Part model, mm, in its own coordinate system. Face numbers are marked on the shaded views. Coordinates: 2 decimals unless noted, no trailing zeros. Order: outer loops, then holes, each group sorted by start corner. A loop starts at its lowest first (then second) coordinate and runs counter-clockwise, first axis right, second up.
Autodesk Fusion 360 part; units mm, degrees
sketch "スケッチ1" plane through (0, 0, 0) normal (0, 0, 1) x (1, 0, 0)
  circle A0 centre (0, 0) radius 50
  circle A1 centre (0, 0) radius 51
  dimension "d1" = 102
ref_plane "作業平面1" through (0, 0, 86) normal (0, 0, 1) x (1, 0, 0)
sketch "スケッチ2" plane through (0, 0, 86) normal (0, 0, 1) x (1, 0, 0)
  circle A0 centre (0, 0) radius 10
  circle A1 centre (0, 0) radius 11
  dimension "d3" = 20
  dimension "d4" = 22
extrude "押し出し1" add sketch "スケッチ1" along normal blind 1 contours A0 | A1
sketch "スケッチ3" plane through (0, 0, 1) normal (0, 0, 1) x (-1, 0, 0)
  circle A0 centre (0, 0) radius 51
  circle A1 centre (0, 0) radius 51
  circle A2 centre (0, 0) radius 50
  dimension "d7" = 100
loft "ロフト1" add profiles "スケッチ3", "スケッチ2" section 1 section 2 contours A0 | A1
loft "ロフト2" cut profiles "スケッチ2", "スケッチ3" section 1 contours A0 section 2 contours A2
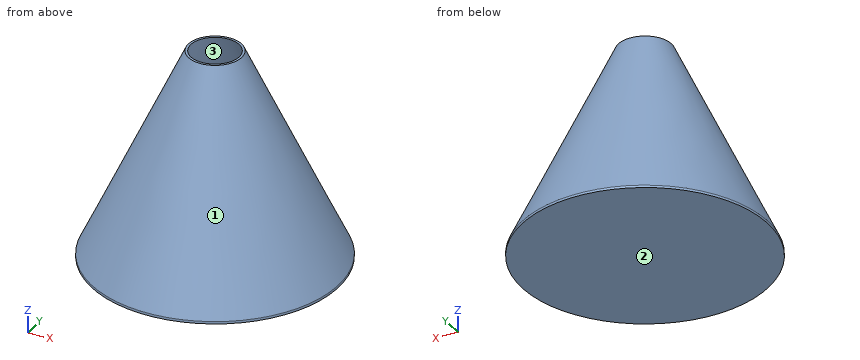
(1) Drop flat-ended pins along their axis: pin 1 (3 mm diameter, centred on x = 14.5, z = 13.5, fed in from +Y); pin 2 (6 mm diameter, centred on x = 22, z = 45, fed in from +Y); pin 3 (6 mm diameter, centred on y = -19, z = 49.5, fed in from +X). Give the stop position or say it passes through.
(2) Probe line 1 (Z direction, x = -26, y = -7.5); line 2 (X direction, y = 24, z = 14); line 3 (X direction, y = 9.5, z = 7). List the from-to ranges inside material, lowest first.
(3) Slice it at C-C, the plane z = 25.5. Give the cut face in (x, y), then the cut area to 3 significant figures.
(4) Slice it at A-A, the plane x = 0. Give the cut face in (y, z), then the cut area to 3 significant figures.
(5) Slice it at B-B, the plane z = 49. Give the cut face in (x, y), then the cut area to 3 significant figures.
(6) Pull direction Y, two halves, no side cores. Call the marked faces 1, 2 and 3: +Y half, -Y half, draft (parallel to the pull), parting line (faces both ways), or undercut.
Here are the results:
1. pin 1: stops at y = 43.61
1. pin 2: stops at y = 24.2
1. pin 3: stops at x = 23.81
2. line 1: z = 0 to 1, 49.75 to 51.87
2. line 2: x = -37.93 to -36.74, 36.74 to 37.93
2. line 3: x = -47.23 to -46.21, 46.21 to 47.23
3. outline: circle Ø78.94 at (0, 0); hole circle Ø76.94 at (0, 0)
3. area: 245 mm2
4. outline: (-51, 0) - (51, 0) - (51, 1) - (11, 86) - (10, 86) - (50, 1) - (-50, 1) - (-10, 86) - (-11, 86) - (-51, 1) - close
4. area: 272 mm2
5. outline: circle Ø56.82 at (0, 0); hole circle Ø54.82 at (0, 0)
5. area: 175 mm2
6. face 1: parting line
6. face 2: draft
6. face 3: undercut
